For this review, take the finished solid that the model builds, in its own axes (mm). Face numbers are marked on the shaded views. A direction names the side the tool comes from. Give positions to 0.01 mm unless a question says otherwise; leave off trailing zeros. Order: outer loops, then holes, each group sorted by start corner. A loop starts at its lowest first (then second) coordinate and runs counter-clockwise, first axis right, second up. Notation, with made-up numbers: (-8.75, -1.75) - (25.25, -1.75) arc R28 cw to (25.25, 23.25) - close; hole circle Ø4 at (20, 83.25). An arc over 180 degrees is marked (long way). Use a Markdown table: item, result. Add a question column.
1) Clearance check with flat-ended pins moving along their axes: P1, Ø2, axis at x = -18.5, y = -23.5, coming from the +Z side; P2, Ø12, axis at x = 8.5, z = 22, coming from the +Y side; P3, Ø7.5, axis at y = 8.5, z = 21, coming from the -X side. State where each tip first meets the part, or that it passes through.
2) We need section C-C on x = 33.5. Write out the cut boundary in (y, z), then the cut area to 3 significant figures.
3) We need section A-A on z = 5.25. Write out the cut boundary in (x, y).
4) Wall thickness on L1, parallel to Y at x = -33.5, z = 0.5; L2, parallel to Y at x = 4, z = 12.5; L3, parallel to X at y = 5, z = 14.5: over which ranges is each line inside the solid? List them lowest first.
5) We need section B-B on y = -24. Write out the cut boundary in (x, z).
6) We need section D-D on x = 13.5. Write out the cut boundary in (y, z), then the cut area to 3 significant figures.
7) Machinability: for the marked faces 4, 5 and 6, which of the approach directions +Z, -Z, +X, -X, +Y, -Y give a long, thin tool a straight path to every point of the face, cutting with its end or side? Answer none if there is none.
8) Mouldability with a two-part tool opening along Y and no side actions: class the marked faces 1, 2 and 3 as released by +Y, released by -Y, zero draft, split by the parting line, or undercut.
Autodesk Inventor part; units mm, degrees
ref_plane "YZ Plane" through (0, 0, 0) normal (1, 0, 0) x (0, 1, 0)
ref_plane "XZ Plane" through (0, 0, 0) normal (0, 1, 0) x (-1, 0, 0)
ref_plane "XY Plane" through (0, 0, 0) normal (0, 0, 1) x (1, 0, 0)
sketch "Эскиз1" plane through (0, 0, 0) normal (0, 0, 1) x (1, 0, 0)
  line L0 (36.5, -27) -> (-36.5, -27)
  line L1 (-36.5, -27) -> (-36.5, 27)
  line L2 (-36.5, 27) -> (36.5, 27)
  line L3 (36.5, 27) -> (36.5, -27)
  line L4 (36.5, -27) -> (-36.5, 27) construction
  line L5 (-36.5, -27) -> (36.5, 27) construction
  circle A0 centre (-33.5, -24) radius 1.6
  circle A1 centre (-33.5, 24) radius 1.6
  circle A2 centre (33.5, 24) radius 1.6
  circle A3 centre (33.5, -24) radius 1.6
  line L6 (-35.1, 24) -> (36.5, 24) construction
  line L7 (-33.5, 27) -> (-33.5, -27) construction
  line L8 (-36.5, -24) -> (36.5, -24) construction
  line L9 (33.5, 27) -> (33.5, -27) construction
  point P0 (0, 0)
  dimension "d6" = 3.2
  dimension "d0" = 73
  dimension "d1" = 54
  dimension "d2" = 3
  dimension "d3" = 3
  dimension "d4" = 3
  dimension "d5" = 3
extrude "Выдавливание1" add sketch "Эскиз1" along normal blind 1
sketch "Эскиз2" plane through (0, 0, 1) normal (0, 0, 1) x (1, 0, 0)
  line L0 (25.5, -2) -> (38.5, -2)
  line L1 (38.5, -2) -> (38.5, -11)
  line L2 (38.5, -11) -> (25.5, -11)
  line L3 (25.5, -11) -> (25.5, -2)
  line L4 (-36.5, -27) -> (36.5, -27)
  line L5 (36.5, -27) -> (36.5, 27)
  point P0 (0, 0)
  dimension "d9" = 13
  dimension "d10" = 9
  dimension "d11" = 16
  dimension "d12" = 2
extrude "Выдавливание2" add sketch "Эскиз2" along normal blind 11.5
sketch "Эскиз3" plane through (0, 0, 1) normal (0, 0, 1) x (1, 0, 0)
  line L0 (-24.5, -28) -> (-1.5, -28)
  line L1 (-1.5, -28) -> (-1.5, -21)
  line L2 (-1.5, -21) -> (-24.5, -21)
  line L3 (-24.5, -21) -> (-24.5, -28)
  line L4 (-36.5, -27) -> (36.5, -27)
  line L5 (-36.5, 27) -> (-36.5, -27)
  line L6 (-14.25, -21) -> (-14.25, -28)
  line L7 (-11.75, -21) -> (-11.75, -28)
  point P0 (0, 0)
  dimension "d15" = 23
  dimension "d16" = 7
  dimension "d17" = 1
  dimension "d18" = 12
  dimension "d21" = 2.5
  dimension "d22" = 10.25
extrude "Выдавливание3" add sketch "Эскиз3" along normal blind 6 contours L3 L4 L6 L0 | L3 L2 L6 L4 | L7 L4 L1 L0 | L7 L2 L1 L4
sketch "Эскиз4" plane through (0, 0, 1) normal (0, 0, 1) x (1, 0, 0)
  line L0 (-33.5, 1) -> (9.5, 1)
  line L1 (9.5, 1) -> (9.5, -16)
  line L2 (9.5, -16) -> (-33.5, -16)
  line L3 (-33.5, -16) -> (-33.5, 1)
  line L4 (-36.5, -27) -> (-24.5, -27)
  line L5 (-36.5, 27) -> (-36.5, -27)
  point P0 (0, 0)
  dimension "d23" = 17
  dimension "d24" = 43
  dimension "d25" = 11
  dimension "d26" = 3
extrude "Выдавливание4" add sketch "Эскиз4" along normal blind 12.5
sketch "Эскиз5" plane through (0, 0, 13.5) normal (0, 0, 1) x (1, 0, 0)
  line L0 (-25, -11) -> (-35, -11)
  line L1 (-35, -11) -> (-35, -4)
  line L2 (-35, -4) -> (-25, -4)
  line L3 (-25, -4) -> (-25, -11)
  line L4 (-25, -11) -> (-35, -4) construction
  line L5 (-35, -11) -> (-25, -4) construction
  line L6 (-35, -7.5) -> (-25, -7.5) construction
  line L7 (-33.5, 1) -> (-33.5, -16)
  point P0 (0, 0)
  point P1 (-30, -7.5)
  point P2 (-33.5, -7.5)
  dimension "d29" = 10
  dimension "d30" = 7
  dimension "d31" = 1.5
extrude "Выдавливание5" add sketch "Эскиз5" along normal blind 4
sketch "Эскиз6" plane through (0, 0, 1) normal (0, 0, 1) x (1, 0, 0)
  line L0 (32, 19) -> (-33, 19)
  line L1 (-33, 19) -> (-33, 4)
  line L2 (-33, 4) -> (32, 4)
  line L3 (32, 4) -> (32, 19)
  line L4 (36.5, 27) -> (-36.5, 27)
  line L5 (-36.5, 27) -> (-36.5, -27)
  point P0 (0, 0)
  dimension "d34" = 15
  dimension "d35" = 65
  dimension "d36" = 8
  dimension "d37" = 3.5
extrude "Выдавливание6" add sketch "Эскиз6" along normal blind 27
equation "\"d3\" = d2"
equation "\"d4\" = d2"
equation "\"d5\" = d2"
equation "\"d22\" = -0.5 * d21 + 0.5 * d15"
properties part number "Плата"
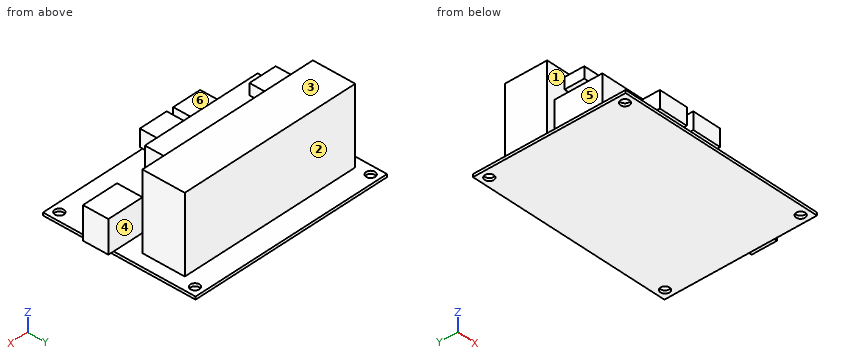
Checked values:
| question | item | result |
|---|---|---|
| 1 | P1 | z = 7 |
| 1 | P2 | y = 19 |
| 1 | P3 | x = -33 |
| 2 | outline | (-27, 0) - (-25.6, 0) - (-25.6, 1) - (-27, 1) - close; (-22.4, 0) - (22.4, 0) - (22.4, 1) - (-2, 1) - (-2, 12.5) - (-11, 12.5) - (-11, 1) - (-22.4, 1) - close; (25.6, 0) - (27, 0) - (27, 1) - (25.6, 1) - close |
| 2 | area | 151 mm² |
| 3 | outline | (-33.5, -16) - (9.5, -16) - (9.5, 1) - (-33.5, 1) - close; (-33, 4) - (32, 4) - (32, 19) - (-33, 19) - close; (-24.5, -28) - (-14.25, -28) - (-14.25, -21) - (-24.5, -21) - close; (-11.75, -28) - (-1.5, -28) - (-1.5, -21) - (-11.75, -21) - close; (25.5, -11) - (38.5, -11) - (38.5, -2) - (25.5, -2) - close |
| 4 | L1 | -27 to -25.6, -22.4 to 22.4, 25.6 to 27 |
| 4 | L2 | -16 to 1, 4 to 19 |
| 4 | L3 | -33 to 32 |
| 5 | outline | (-36.5, 0) - (-35.1, 0) - (-35.1, 1) - (-36.5, 1) - close; (-31.9, 0) - (31.9, 0) - (31.9, 1) - (-1.5, 1) - (-1.5, 7) - (-11.75, 7) - (-11.75, 1) - (-14.25, 1) - (-14.25, 7) - (-24.5, 7) - (-24.5, 1) - (-31.9, 1) - close; (35.1, 0) - (36.5, 0) - (36.5, 1) - (35.1, 1) - close |
| 6 | outline | (-27, 0) - (27, 0) - (27, 1) - (19, 1) - (19, 28) - (4, 28) - (4, 1) - (-27, 1) - close |
| 6 | area | 459 mm² |
| 7 | face 4 | +Z, +X |
| 7 | face 5 | -X, +Y, -Y |
| 7 | face 6 | +Z, +X, -X, -Y |
| 8 | face 1 | undercut |
| 8 | face 2 | released by +Y |
| 8 | face 3 | zero draft |
